Geometry check sheet. Reference: the model listing, model coordinates, mm. Face numbers are marked on the shaded views. Give positions to 0.01 mm unless a question says otherwise; leave off trailing zeros. Order: outer loops, then holes, each group sorted by start corner. A loop starts at its lowest first (then second) coordinate and runs counter-clockwise, first axis right, second up. Notation, with made-up numbers: M 14,50.5 L 43,50.5 A26 ccw 43,70.5 Z; hole C -9,63 d10. An arc over 180 degrees is marked long. Put each result on its own line as item: value. Start each with the question number.
Q1. Material ranges on L1, parallel to X at y = 8, z = 38; L2, parallel to Z at x = -33, y = -15.5; L3, parallel to Y at x = -249.5, z = 15.5, recorded low to high.
Q2. Go/stop test with flat-tipped pins: pin 1 (1 mm diameter, centred on x = -131.5, z = -21, fed in from -Y); pin 2 (4 mm diameter, centred on y = -7, z = -37.5, fed in from -X); pin 3 (6 mm diameter, centred on x = 173.5, y = -4.5, fed in from +Z). Record where each tip stops, or that it passes through.
Q3. Section check A-A on y = 19.5. Record the cut outline in (x, z).
Q4. Mould release check, pull along X, two halves, no side actions. Record for the marked faces 1 and 2: +X half, -X half, draft (parallel to the pull), parting line (faces both ways), or undercut.
Q5. Section check D-D on y = -41.5. Record the cut outline in (x, z).
```python
from build123d import *

# Parameters (mm, degrees)
BASE_FLANGE1_DEPTH      = 304.8
EDGE_FLANGE1_DEPTH      = 85.725
EDGE_FLANGE1_BEND_DEPTH = 85.725


# Sheet-metal steps are written as plain solids
with BuildPart() as part:
    # Sketch1 → Base-Flange1 (new, symmetric)
    with BuildSketch(Plane(origin=(0, 0, 0), x_dir=(0, 0, -1), z_dir=(1, 0, 0))):
        with BuildLine():
            Line((-57.15, -50.8), (-57.15, -14.2875))
            ThreePointArc((-57.15, -14.2875), (-52.965288136, -4.184711864), (-42.8625, 0))
            Line((-42.8625, 0), (42.8625, 0))
            ThreePointArc((42.8625, 0), (52.965288136, -4.184711864), (57.15, -14.2875))
            Line((57.15, -14.2875), (57.15, -50.8))
            Line((57.15, -50.8), (50.8, -50.8))
            Line((50.8, -50.8), (50.8, -14.2875))
            ThreePointArc((50.8, -14.2875), (48.475160076, -8.674839924), (42.8625, -6.35))
            Line((42.8625, -6.35), (-42.8625, -6.35))
            ThreePointArc((-42.8625, -6.35), (-48.475160076, -8.674839924), (-50.8, -14.2875))
            Line((-50.8, -14.2875), (-50.8, -50.8))
            Line((-50.8, -50.8), (-57.15, -50.8))
        make_face()
    extrude(amount=BASE_FLANGE1_DEPTH, both=True)

    # Edge-Flange1 section (across the edge) → Edge-Flange1 (add)
    with BuildSketch(Plane(origin=(312.7375, 0, 42.8625), x_dir=(-1, 0, 0), z_dir=(0, 0, -1))):
        with BuildLine():
            Line((-6.35, 7.9375), (-6.35, 44.45))
            Line((-6.35, 44.45), (0, 44.45))
            Line((0, 44.45), (0, 7.9375))
            ThreePointArc((0, 7.9375), (2.324839924, 2.324839924), (7.9375, 0))
            Line((7.9375, 0), (7.9375, -6.35))
            ThreePointArc((7.9375, -6.35), (-2.165288136, -2.165288136), (-6.35, 7.9375))
        make_face()
    extrude(amount=EDGE_FLANGE1_DEPTH)

    # Edge-Flange1 section 2 (across the edge) → Edge-Flange1 bend (add)
    with BuildSketch(Plane(origin=(-312.7375, 0, -42.8625), x_dir=(1, 0, 0), z_dir=(0, 0, 1))):
        with BuildLine():
            Line((-6.35, 7.9375), (-6.35, 44.45))
            Line((-6.35, 44.45), (0, 44.45))
            Line((0, 44.45), (0, 7.9375))
            ThreePointArc((0, 7.9375), (2.324839924, 2.324839924), (7.9375, 0))
            Line((7.9375, 0), (7.9375, -6.35))
            ThreePointArc((7.9375, -6.35), (-2.165288136, -2.165288136), (-6.35, 7.9375))
        make_face()
    extrude(amount=EDGE_FLANGE1_BEND_DEPTH)


solid = part.part
```
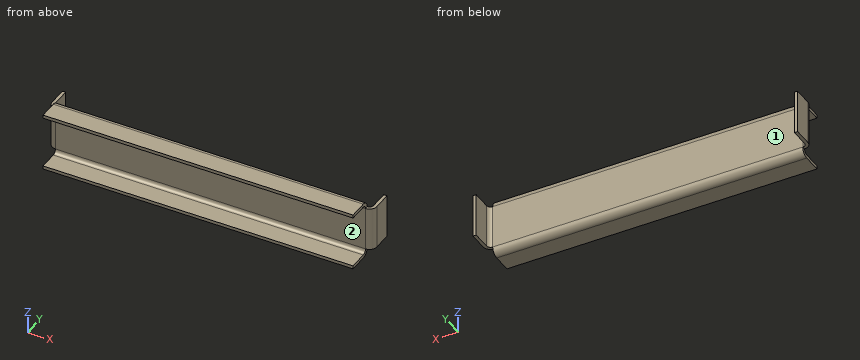
Results found:
1. L1: x = -319.09 to -312.74, 312.74 to 319.09
1. L2: z = -57.15 to -50.8, 50.8 to 57.15
1. L3: y = -6.35 to 0
2. pin 1: stops at y = -6.35
2. pin 2: stops at x = -310.86
2. pin 3: stops at z = 55.43
3. outline: M -319.09,-42.86 L -312.74,-42.86 L -312.74,42.86 L -319.09,42.86 Z; M 312.74,-42.86 L 319.09,-42.86 L 319.09,42.86 L 312.74,42.86 Z
4. face 1: undercut
4. face 2: draft
5. outline: M -304.8,-57.15 L 304.8,-57.15 L 304.8,-50.8 L -304.8,-50.8 Z; M -304.8,50.8 L 304.8,50.8 L 304.8,57.15 L -304.8,57.15 Z
